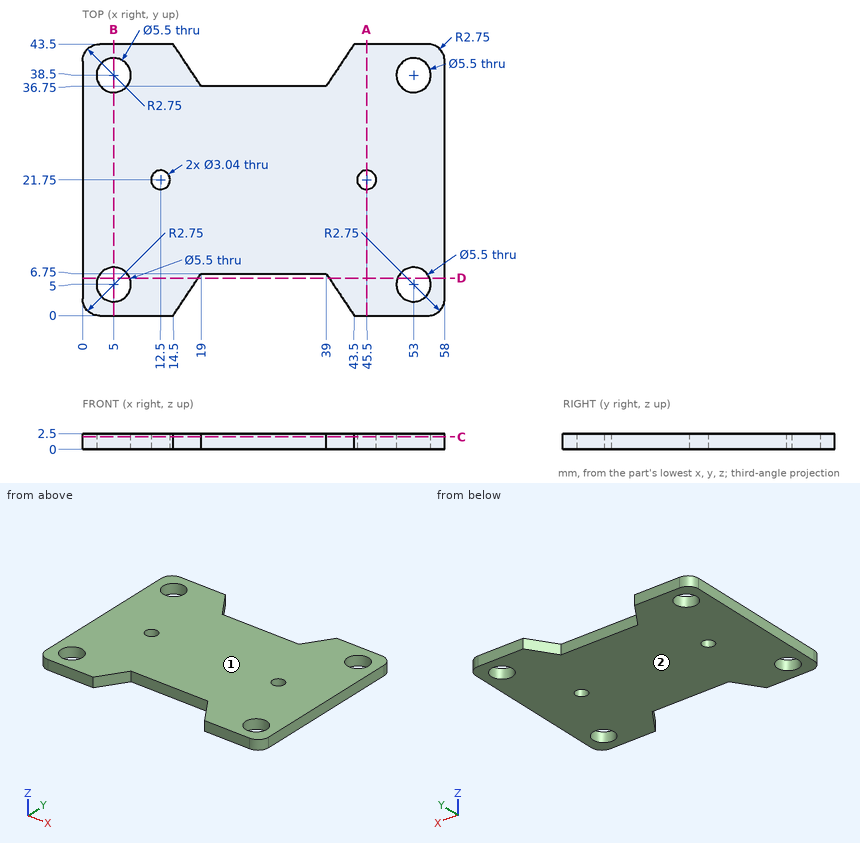
Check sheet for the drawn part. Datum: minimum x, y, z corner. Units: mm. Round coordinates to 2 decimals unless told otherwise and drop trailing zeros. Order: outer loops, then holes, each group sorted by start corner. A loop starts at its lowest first (then second) coordinate and runs counter-clockwise, first axis right, second up. Notation, with made-up numbers: (37.5, 62) -> (58.5, 62) arc R23 ccw to (58.5, 85) -> close; hole circle Ø5 at (-23.75, -38.75). An arc over 180 degrees is marked (long way). Put each result on its own line as item: value. Start each with the question number.
(1) Section check B-B (x = 5). Enter the section's corners in (y, z).
(2) Section check D-D (y = 6). Enter the section's corners in (x, z), then the cut area to 3 significant figures.
(3) Section check A-A (x = 45.5). Enter the section's corners in (y, z), then the cut area to 3 significant figures.
(4) Material ranges on line 1 along Y through (x, z) = (5, 1.2); line 2 along Y through (x, z) = (12.5, 0.6); line 3 along Y through (x, z) = (54, 1.7), recorded low to high.
(5) Draft check along Z on the marked faces 1 and 2. Enter one of: +Z half, -Z half, draft (parallel to the pull), parting line (faces both ways), or undercut.
(6) Section check C-C (z = 2). Enter the section's corners in (x, y).
Completed:
1. outline: (0, 0) -> (2.25, 0) -> (2.25, 2.5) -> (0, 2.5) -> close; (7.75, 0) -> (35.75, 0) -> (35.75, 2.5) -> (7.75, 2.5) -> close; (41.25, 0) -> (43.5, 0) -> (43.5, 2.5) -> (41.25, 2.5) -> close
2. outline: (0, 0) -> (2.44, 0) -> (2.44, 2.5) -> (0, 2.5) -> close; (7.56, 0) -> (18.5, 0) -> (18.5, 2.5) -> (7.56, 2.5) -> close; (39.5, 0) -> (50.44, 0) -> (50.44, 2.5) -> (39.5, 2.5) -> close; (55.56, 0) -> (58, 0) -> (58, 2.5) -> (55.56, 2.5) -> close
2. area: 66.9 mm2
3. outline: (0, 0) -> (20.23, 0) -> (20.23, 2.5) -> (0, 2.5) -> close; (23.27, 0) -> (43.5, 0) -> (43.5, 2.5) -> (23.27, 2.5) -> close
3. area: 101 mm2
4. line 1: y = 0 to 2.25, 7.75 to 35.75, 41.25 to 43.5
4. line 2: y = 0 to 20.23, 23.27 to 43.5
4. line 3: y = 0 to 2.44, 7.56 to 35.94, 41.06 to 43.5
5. face 1: +Z half
5. face 2: -Z half
6. outline: (0, 2.75) arc R2.75 ccw to (2.75, 0) -> (14.5, 0) -> (19, 6.75) -> (39, 6.75) -> (43.5, 0) -> (55.25, 0) arc R2.75 ccw to (58, 2.75) -> (58, 40.75) arc R2.75 ccw to (55.25, 43.5) -> (43.5, 43.5) -> (39, 36.75) -> (19, 36.75) -> (14.5, 43.5) -> (2.75, 43.5) arc R2.75 ccw to (0, 40.75) -> close; hole circle Ø5.5 at (5, 5); hole circle Ø5.5 at (5, 38.5); hole circle Ø3.04 at (12.5, 21.75); hole circle Ø3.04 at (45.5, 21.75); hole circle Ø5.5 at (53, 5); hole circle Ø5.5 at (53, 38.5)
